```python
from build123d import *

# Parameters (mm, degrees)
F0_W          = 30
F0_H          = 30
F1_DEPTH      = 15
F1_DEPTH_BACK = 15
F2_R          = 4
F3_DEPTH      = 1
F4_R          = 3.5
F5_DEPTH      = 2
F6_R          = 3.5
F7_DEPTH      = 2
F8_R          = 3.5
F9_DEPTH      = 2
F10_R         = 3.5
F11_DEPTH     = 2
F12_R         = 3.5
F13_DEPTH     = 2
F14_R         = 1


with BuildPart() as f1:
    # F0 (on Top) → F1 (new body, two sides)
    with BuildSketch(Plane.XY) as f1_sk:
        Rectangle(F0_W, F0_H)
    extrude(amount=F1_DEPTH)
    extrude(f1_sk.sketch, amount=-F1_DEPTH_BACK)

    # F2 (on face) → F3 (cut)
    with BuildSketch(Plane.XZ.offset(15)):
        Circle(F2_R)
    extrude(amount=-F3_DEPTH, mode=Mode.SUBTRACT)

    # F4 (on face) → F5 (cut)
    with BuildSketch(Plane(origin=(0, 15, 0), x_dir=(-1, 0, 0), z_dir=(0, 1, 0))):
        with Locations((-6, 8.5)):
            Circle(F4_R)
        with Locations((6, 8.5)):
            Circle(F4_R)
        with Locations((6, 0)):
            Circle(F4_R)
        with Locations((-6, 0)):
            Circle(F4_R)
        with Locations((6, -8.5)):
            Circle(F4_R)
        with Locations((-6, -8.5)):
            Circle(F4_R)
    extrude(amount=-F5_DEPTH, mode=Mode.SUBTRACT)

    # F6 (on face) → F7 (cut)
    with BuildSketch(Plane(origin=(0, 0, -15), x_dir=(1, 0, 0), z_dir=(0, 0, -1))):
        with Locations((0, -7.5)):
            Circle(F6_R)
        with Locations((0, 7.5)):
            Circle(F6_R)
    extrude(amount=-F7_DEPTH, mode=Mode.SUBTRACT)

    # F8 (on face) → F9 (cut)
    with BuildSketch(Plane.XY.offset(15)):
        with Locations((-7.5, -7.5)):
            Circle(F8_R)
        with Locations((-7.5, 7.5)):
            Circle(F8_R)
        Circle(F8_R)
        with Locations((7.5, 7.5)):
            Circle(F8_R)
        with Locations((7.5, -7.5)):
            Circle(F8_R)
    extrude(amount=-F9_DEPTH, mode=Mode.SUBTRACT)

    # F10 (on face) → F11 (cut)
    with BuildSketch(Plane(origin=(-15, 0, 0), x_dir=(0, -1, 0), z_dir=(-1, 0, 0))):
        with Locations((7.5, -7.5)):
            Circle(F10_R)
        with Locations((-7.5, -7.5)):
            Circle(F10_R)
        with Locations((7.5, 7.5)):
            Circle(F10_R)
        with Locations((-7.5, 7.5)):
            Circle(F10_R)
    extrude(amount=-F11_DEPTH, mode=Mode.SUBTRACT)

    # F12 (on face) → F13 (cut)
    with BuildSketch(Plane.YZ.offset(15)):
        with Locations((0, 8.67)):
            Circle(F12_R)
        with Locations((-7.483315, -4.33)):
            Circle(F12_R)
        with Locations((7.516673, -4.310741)):
            Circle(F12_R)
    extrude(amount=-F13_DEPTH, mode=Mode.SUBTRACT)

    # F14
    f14_edges = [f1.edges().sort_by_distance(p)[0] for p in [
        (0, 15, 15),
        (15, 15, 0),
        (0, 15, -15),
        (-15, 15, 0),
        (-15, 0, -15),
        (15, 0, -15),
        (15, -15, 0),
        (15, 0, 15),
        (-15, 0, 15),
        (0, -15, 15),
        (0, -15, -15),
    ]]
    fillet(f14_edges, radius=F14_R)


solid = f1.part
```
The model under review builds one solid part; all positions refer to its coordinate system, in mm. A direction names the side the tool comes from. Give positions to 0.01 mm unless a question says otherwise; leave off trailing zeros. Write each loop counter-clockwise with the first axis right and the second up, starting at its lowest first coordinate (ties: lowest second). Pieces come first, ordered by that corner, then holes. Notation, with made-up numbers: (41.5, 35.25) - (97.5, 35.25) arc R9 cw to (97.5, 49.25) - close; hole circle Ø5 at (11, 12). An arc over 180 degrees is marked (long way). Answer in a Markdown table with one row per item. Add a question column.
1. We need section A-A on y = 0. Write out the cut boundary in (x, z).
2. Insertion check: P1, Ø3.5, axis at x = 7.5, y = 6, coming from the +Z side; P2, Ø1, axis at x = -7, z = 0.5, coming from the +Y side; P3, Ø4, axis at y = 7.5, z = 7.5, coming from the -X side. Each pin has a flat end and moves straight along its axis. Give the tip position at first contact, or say it passes through.
3. We need section B-B on z = 0. Write out the cut boundary in (x, y).
4. Tool access review of faces 1 (the flat face through (-8, -7, 13)), 2 (the cylindrical face through (-14.014, -4.003, -7.346)), 3 (the flat face through (-6, 13, 9)), 4 (the flat face through (0, -8, -13)): name each direction out of +Z, -Z, +X, -X, +Y, -Y from which nothing blocks a thin tool from reaching the whole face with its end or side.
5. We need section C-C on x = 7.5. Write out the cut boundary in (y, z).
6. Wall thickness on line 1 along Z through (x, y) = (6, 13.4); line 2 along Z through (x, y) = (-14, 7.5): over which ranges is each line inside the solid? List them lowest first. Write a range as [from, to].
7. We need section D-D on x = 0. Write out the cut boundary in (y, z), then the cut area to 3 significant figures.
8. Draft analysis for pull direction Y (two halves, no side actions). For faces 5 (the cylindrical face through (6.759, 14.014, 5.083)), 6 (the flat face through (-8, 8, 13)), 7 (the flat face through (-6, 13, -8)), state which applies: +Y half, -Y half, draft (parallel to the pull), parting line (faces both ways), or undercut.
Ans:
| question | item | result |
|---|---|---|
| 1 | outline | (-15, -14) arc R1 ccw to (-14, -15) - (14, -15) arc R1 ccw to (15, -14) - (15, 5.17) - (13, 5.17) - (13, 12.17) - (15, 12.17) - (15, 14) arc R1 ccw to (14, 15) - (3.5, 15) - (3.5, 13) - (-3.5, 13) - (-3.5, 15) - (-14, 15) arc R1 ccw to (-15, 14) - close |
| 2 | P1 | stops at z = 13 |
| 2 | P2 | stops at y = 13 |
| 2 | P3 | stops at x = -13 |
| 3 | outline | (-15, -15) - (-4, -15) - (-4, -14) - (4, -14) - (4, -15) - (14, -15) arc R1 ccw to (15, -14) - (15, 14) arc R1 ccw to (14, 15) - (9.5, 15) - (9.5, 13) - (2.5, 13) - (2.5, 15) - (-2.5, 15) - (-2.5, 13) - (-9.5, 13) - (-9.5, 15) - (-14, 15) arc R1 ccw to (-15, 14) - close |
| 4 | face 1 | +Z |
| 4 | face 2 | -X |
| 4 | face 3 | +Y |
| 4 | face 4 | -Z |
| 5 | outline | (-15, -14) arc R1 ccw to (-14, -15) - (14, -15) arc R1 ccw to (15, -14) - (15, -11.66) - (13, -11.66) - (13, -5.34) - (15, -5.34) - (15, -3.16) - (13, -3.16) - (13, 3.16) - (15, 3.16) - (15, 5.34) - (13, 5.34) - (13, 11.66) - (15, 11.66) - (15, 14) arc R1 ccw to (14, 15) - (11, 15) - (11, 13) - (4, 13) - (4, 15) - (-4, 15) - (-4, 13) - (-11, 13) - (-11, 15) - (-14, 15) arc R1 ccw to (-15, 14) - close |
| 6 | line 1 | z = [-15, -12], [-5, -3.5], [3.5, 5], [12, 15] |
| 6 | line 2 | z = [-15, -11], [-4, 4], [11, 15] |
| 7 | outline | (-15, -14) arc R1 ccw to (-14, -15) - (-11, -15) - (-11, -13) - (-4, -13) - (-4, -15) - (4, -15) - (4, -13) - (11, -13) - (11, -15) - (14, -15) arc R1 ccw to (15, -14) - (15, 14) arc R1 ccw to (14, 15) - (3.5, 15) - (3.5, 13) - (-3.5, 13) - (-3.5, 15) - (-14, 15) arc R1 ccw to (-15, 14) - (-15, 4) - (-14, 4) - (-14, -4) - (-15, -4) - close |
| 7 | area | 849 mm^2 |
| 8 | face 5 | draft |
| 8 | face 6 | undercut |
| 8 | face 7 | +Y half |
